Part model, mm, in its own coordinate system. Face numbers are marked on the shaded views. Give positions to 0.01 mm unless a question says otherwise; leave off trailing zeros. Loops run counter-clockwise (first coordinate to the right, second up) from the corner with the lowest first, then second, coordinate; pieces in that order, holes last. Notation, with made-up numbers: (65.25, 53.25) -> (79.25, 53.25) arc R14 ccw to (79.25, 80.25) -> close; hole circle Ø4 at (-4, 14). An arc over 180 degrees is marked (long way). One line per question, with ' | ' between items.
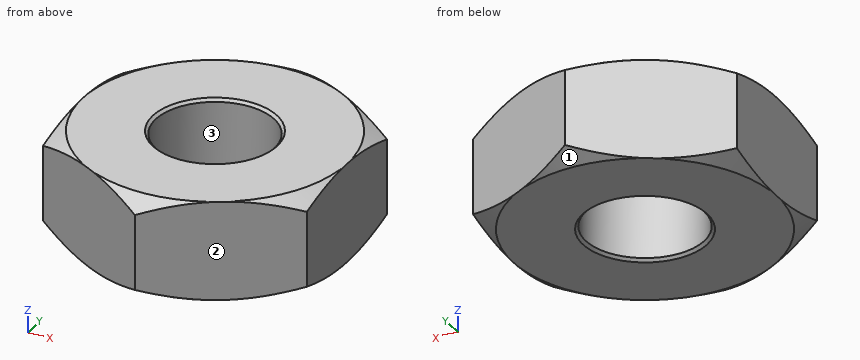
```python
from build123d import *

# Parameters (mm, degrees)
BOSS_EXTRUDE1_START = -1.190625
SKETCH3_R           = 1.4224
BOSS_EXTRUDE1_DEPTH = 2.38125


# Read off the part's stored shape, not the designer's step: Cut-Revolve1
with BuildPart() as part:
    # Sketch3 → Boss-Extrude1 (new body)
    with BuildSketch(Plane.XY.offset(BOSS_EXTRUDE1_START)):
        Polygon((-3.175, 1.833087105), (-3.175, -1.833087105), (0, -3.666174209), (3.175, -1.833087105), (3.175, 1.833087105), (0, 3.666174209), align=None)
        with Locations(Location((0, 0, 0), (0, 0, 180))):
            Circle(SKETCH3_R, mode=Mode.SUBTRACT)
    extrude(amount=BOSS_EXTRUDE1_DEPTH)

    # Cut-Revolve1 outline → Cut-Revolve1 (revolve, cut)
    with BuildSketch(Plane.XZ):
        Polygon((3.66617421, -0.907045438), (3.174999964, -1.190625021), (3.666174217, -1.190625256), align=None)
        Polygon((3.175, 1.190625), (3.66617421, 0.907045438), (3.666174217, 1.190625256), align=None)
    revolve(axis=Axis((0, 0, 0), (0, 0, 1)), mode=Mode.SUBTRACT)

    # Sketch9 → Cut-Revolve2 (revolve, cut)
    with BuildSketch(Plane(origin=(0, 0, 0), x_dir=(0, 0, -1), z_dir=(1, 0, 0)), mode=Mode.PRIVATE) as cut_revolve2_sk:
        Polygon((-1.121884234, 1.4224), (-1.7859375, 2.086453266), (-1.7859375, 1.4224), (-1.7859375, 0), (-1.121884234, 0), (-0.640698869, 0), (-0.640698869, 0.941214635), align=None)
        Polygon((1.7859375, 2.086453266), (1.7859375, 1.4224), (1.7859375, 0), (1.121884234, 0), (0.640698869, 0), (0.640698869, 0.941214635), (1.121884234, 1.4224), align=None)
    revolve(cut_revolve2_sk.sketch.rotate(Axis((0, 0, 1.190625), (0, 0, -1)), 270), axis=Axis((0, 0, 1.190625), (0, 0, -1)), mode=Mode.SUBTRACT)


solid = part.part
```
1) Saw through at A-A (z = -0.1). Give the cut face in (x, y) (3 decimals).
Found:
outline: (-3.175, -1.833) -> (0, -3.666) -> (3.175, -1.833) -> (3.175, 1.833) -> (0, 3.666) -> (-3.175, 1.833) -> close; hole circle Ø2.845 at (0, 0)
2) Drill centre lines: line 1 (X direction, y = 1.25, z = 0) (3 decimals); line 2 (Y direction, x = 1, z = 0.95); line 3 (Y direction, x = 0.25, z = 0.6). Where is each one in solid material? Low to high.
Found:
line 1: -3.175 to -0.679, 0.679 to 3.175 | line 2: -3.09 to -1.01, 1.01 to 3.09 | line 3: -3.52 to -1.4, 1.4 to 3.52
3) Saw through at B-B (z = -1). Give the cut face in (x, y) (3 decimals).
Found:
outline: (-3.175, -1.485) arc R3.505 ccw to (-2.874, -2.007) -> (-0.301, -3.492) arc R3.505 ccw to (0.301, -3.492) -> (2.874, -2.007) arc R3.505 ccw to (3.175, -1.485) -> (3.175, 1.485) arc R3.505 ccw to (2.874, 2.007) -> (0.301, 3.492) arc R3.505 ccw to (-0.301, 3.492) -> (-2.874, 2.007) arc R3.505 ccw to (-3.175, 1.485) -> close; hole circle Ø2.845 at (0, 0)
4) Pull direction X, two halves, no side cores. Call the marked faces 1, 2 and 3: pulls with the +X half, pulls with the -X half, needs draft (parallel to the pull), parting line crosses it, or undercut.
Found:
face 1: parting line crosses it | face 2: pulls with the +X half | face 3: undercut
